from build123d import *

# Parameters (mm, degrees)
SKETCH1_R           = 8
SKETCH1_W           = 5.5
SKETCH1_H           = 3.7
BOSS_EXTRUDE1_DEPTH = 5
CUT_EXTRUDE1_DEPTH  = 13.369316877
CIRPATTERN1_COUNT   = 6
FILLET1_R           = 10


with BuildPart() as part:
    # Sketch1 → Boss-Extrude1 (new body)
    with BuildSketch(Plane.XY):
        Circle(SKETCH1_R)
        Rectangle(SKETCH1_W, SKETCH1_H, mode=Mode.SUBTRACT)
    extrude(amount=BOSS_EXTRUDE1_DEPTH)

    # Sketch2 → Cut-Extrude1 (cut, through all)
    with BuildSketch(Plane.XY):
        Polygon((-7.331932906, 22.221764399), (0, 24.952212466), (7.331932906, 22.221764399), (3.798424573, 7.040736522), (3.120998591, 6.924019842), (1.330058439, 5.723612136), (0.501497444, 4.50257488), (-0.501497444, 4.50257488), (-1.330058439, 5.723612136), (-3.120998591, 6.924019842), (-3.798424573, 7.040736522), align=None)
    cut_extrude1 = extrude(amount=CUT_EXTRUDE1_DEPTH, mode=Mode.SUBTRACT)

    # CirPattern1: Cut-Extrude1 ×6 about axis
    cirpattern1_axis = Axis((0, 0, 0), (0, 0, 1))
    for i in range(1, CIRPATTERN1_COUNT):
        add(cut_extrude1.rotate(cirpattern1_axis, i * 360 / CIRPATTERN1_COUNT), mode=Mode.SUBTRACT)

    # Fillet1
    # the kernel refuses this fillet: 10 mm, written as the material it takes off along each edge
    with BuildSketch(Plane(origin=(-1.330058439, -5.723612136, -4.777865205), x_dir=(0.5615014183372642, 0.8274757743917586, 0), z_dir=(0, 0, 1)), Plane(origin=(5.621822731, 1.709941671, -4.777865205), x_dir=(-0.997365750808096, 0.07253660534518461, 0), z_dir=(0, 0, 1)), Plane(origin=(4.291764291, -4.013670465, -4.777865205), x_dir=(-0.43586433247083195, 0.9000123797369435, 0), z_dir=(0, 0, 1)), Plane(origin=(-5.621822731, -1.709941671, -4.777865205), x_dir=(0.997365750808096, -0.07253660534518423, 0), z_dir=(0, 0, 1)), Plane(origin=(-4.291764291, 4.013670465, -4.777865205), x_dir=(0.43586433247083256, -0.900012379736943, 0), z_dir=(0, 0, 1)), Plane(origin=(1.330058439, 5.723612136, -4.777865205), x_dir=(-0.561501418337264, -0.8274757743917588, 0), z_dir=(0, 0, 1))) as fillet1_piece_1:
        with BuildLine():
            CenterArc((1.975419419, 9.987502063), FILLET1_R, 247.992328485, 19.142820558)
            Line((-1.771887917, 0.716165173), (-1.846834064, 0.530738436))
            Line((-1.846834064, 0.530738436), (-0.074946147, -0.185426738))
            Line((-0.074946147, -0.185426738), (0, -0.2))
            ThreePointArc((0, -0.2), (0.737808461, -0.2), (1.465620873, -0.199750041))
            Line((1.465620873, -0.199750041), (1.475616922, 0))
        make_face()
    extrude(amount=14.55573041, mode=Mode.SUBTRACT)
    with BuildSketch(Plane(origin=(5.621822731, -1.709941671, -4.777865205), x_dir=(0.8975096924716217, 0.44099473003596645, 0), z_dir=(0, 0, 1)), Plane(origin=(1.330058439, -5.723612136, -4.777865205), x_dir=(0.8306674853820185, -0.5567688288052, 0), z_dir=(0, 0, 1)), Plane(origin=(-4.291764291, -4.013670465, -4.777865205), x_dir=(-0.06684220708960342, -0.9977635588411669, 0), z_dir=(0, 0, 1)), Plane(origin=(-5.621822731, 1.709941671, -4.777865205), x_dir=(-0.8975096924716216, -0.44099473003596684, 0), z_dir=(0, 0, 1)), Plane(origin=(4.291764291, 4.013670465, -4.777865205), x_dir=(0.06684220708960296, 0.9977635588411669, 0), z_dir=(0, 0, 1)), Plane(origin=(-1.330058439, 5.723612136, -4.777865205), x_dir=(-0.8306674853820185, 0.5567688288052001, 0), z_dir=(0, 0, 1))) as fillet1_piece_2:
        with BuildLine():
            CenterArc((1.911146082, 10), FILLET1_R, 250.857179442, 19.142820558)
            Line((-1.368094161, 0.552959012), (-1.433678966, 0.364018192))
            ThreePointArc((-1.433678966, 0.364018192), (-0.758993227, 0.091052768), (-0.074946147, -0.185426738))
            Line((-0.074946147, -0.185426738), (0, -0.2))
            Line((0, -0.2), (1.911146082, -0.2))
            Line((1.911146082, -0.2), (1.911146082, 0))
        make_face()
    extrude(amount=14.55573041, mode=Mode.SUBTRACT)


solid = part.part
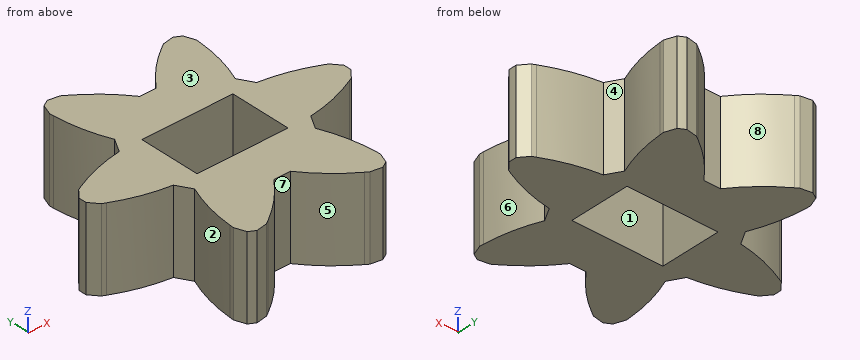
Read the model definition and answer for the solid it produces. Units are mm, in the model's axes. Face numbers are marked on the shaded views. A direction names the side the tool comes from. Round coordinates to 2 decimals unless told otherwise and drop trailing zeros. Order: outer loops, then holes, each group sorted by start corner. A loop starts at its lowest first (then second) coordinate and runs counter-clockwise, first axis right, second up.
1) The part is cut by section B-B on x = 2.5. Write down the section's boundary in (y, z), plus the area to 3 significant figures.
2) The mould has two halves that part along Y. Classify the marked faces 6, 7 and 8: released by +Y, released by -Y, zero draft, split by the parting line, or undercut.
3) Flat-ended cylindrical pins translate along their axes: pin 1 (1.5 mm diameter, centred on x = 0, z = 2.5, fed in from +Y); pin 2 (0.5 mm diameter, centred on x = 0, z = 2, fed in from +Y); pin 3 (2 mm diameter, centred on x = -5.5, z = 1.5, fed in from -Y). Find the tip coordinate at first contact, or state that the pin passes through.
4) Straight lines are drawn through the part: L1, parallel to X at y = 0, z = 4.3; L2, parallel to X at y = 6.5, z = 3.45; L3, parallel to Y at x = 1.75, z = 2.15. For each, find the intervals that lie inside material, in ascending order.
5) The part is cut by section A-A on y = 4.75. Write down the section's boundary in (x, z), plus the area to 3 significant figures.
6) For the marked faces 1, 2, 3, 4 and 5, determine the directions among +Z, -Z, +X, -X, +Y, -Y from which every point of the face is accessible in a straight line to the end or side of a thin tool.
7) The part is cut by section C-C on x = -5.25. Write down the section's boundary in (y, z), plus the area to 3 significant figures.
8) The part is cut by section D-D on y = -3. Write down the section's boundary in (x, z), plus the area to 3 significant figures.
Resolved:
1. outline: (-6.49, 0) - (-1.85, 0) - (-1.85, 5) - (-6.49, 5) - close; (1.85, 0) - (6.49, 0) - (6.49, 5) - (1.85, 5) - close
1. area: 46.4 mm2
2. face 6: undercut
2. face 7: released by -Y
2. face 8: released by +Y
3. pin 1: stops at y = 4.82
3. pin 2: stops at y = 4.5
3. pin 3: stops at y = -1.77
4. L1: x = -8 to -2.75, 2.75 to 8
4. L2: x = -4.31 to -2.51, 2.51 to 4.31
4. L3: y = -5.87 to -1.85, 1.85 to 5.87
5. outline: (-4.27, 0) - (-0.69, 0) - (-0.69, 5) - (-4.27, 5) - close; (0.69, 0) - (4.27, 0) - (4.27, 5) - (0.69, 5) - close
5. area: 35.8 mm2
6. face 1: +Z, -Z
6. face 2: +Z, -Z, -X
6. face 3: +Z, +X, -X, +Y, -Y
6. face 4: +Z, -Z, +X
6. face 5: +Z, -Z, -Y
7. outline: (-1.62, 0) - (1.62, 0) - (1.62, 5) - (-1.62, 5) - close
7. area: 16.2 mm2
8. outline: (-3.78, 0) - (3.78, 0) - (3.78, 5) - (-3.78, 5) - close
8. area: 37.8 mm2
